For this review, take the finished solid that the model builds, in its own axes (mm). Face numbers are marked on the shaded views. A direction names the side the tool comes from. Give positions to 0.01 mm unless a question says otherwise; leave off trailing zeros. Write each loop counter-clockwise with the first axis right and the second up, starting at its lowest first coordinate (ties: lowest second). Pieces come first, ordered by that corner, then holes. Notation, with made-up numbers: (16, 61) -> (48, 61) arc R22 cw to (48, 69) -> close; hole circle Ø2 at (66, -20). An arc over 180 degrees is marked (long way). Write item = value, one per line.
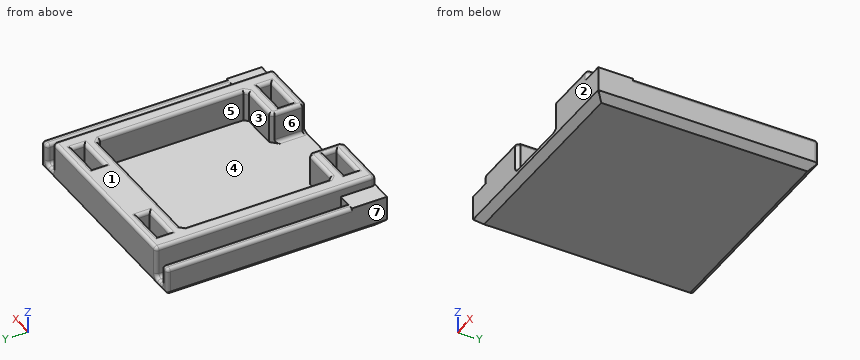
```python
from build123d import *

# Parameters (mm, degrees)
BOSS_EXTRU_2_DEPTH      = 9
ESQUISSE3_W             = 51.8612703
ESQUISSE3_H             = 63
BOSS_EXTRU_3_DEPTH      = 3
ESQUISSE4_W             = 10
ESQUISSE4_H             = 3.4
ENL_V_MAT_EXTRU_1_DEPTH = 7
ESQUISSE5_W             = 3.2
ESQUISSE5_H             = 3
BOSS_EXTRU_4_DEPTH      = 63
CHANFREIN1_SIZE         = 1
CHANFREIN2_SIZE         = 2
CONG_1_R                = 1
CONG_2_R                = 1
CHANFREIN4_SIZE         = 1
CONG_4_R                = 1
CONG_5_R                = 1
ESQUISSE6_W             = 6.7
ESQUISSE6_H             = 1
BOSS_EXTRU_5_DEPTH      = 10


with BuildPart() as part:
    # Esquisse2 → Boss.-Extru.2 (new body)
    with BuildSketch(Plane.XY):
        Polygon((-9.3, -31.5), (-9.3, -21.5), (-21.5, -21.5), (-21.5, 21.5), (21.5, 21.5), (21.5, -21.5), (9.3, -21.5), (9.3, -31.5), (25.93063515, -31.5), (25.93063515, 31.5), (-25.93063515, 31.5), (-25.93063515, -31.5), align=None)
    extrude(amount=BOSS_EXTRU_2_DEPTH)

    # Esquisse3 → Boss.-Extru.3 (add)
    with BuildSketch(Plane(origin=(0, 0, 0), x_dir=(-1, 0, 0), z_dir=(0, 0, -1))):
        Rectangle(ESQUISSE3_W, ESQUISSE3_H)
    extrude(amount=BOSS_EXTRU_3_DEPTH)

    # Esquisse4 → Enlèv. mat.-Extru.1 (cut)
    with BuildSketch(Plane.XY.offset(9)):
        with Locations((-16.5, -26.695538472)):
            Rectangle(ESQUISSE4_W, ESQUISSE4_H)
        with Locations((16.5, -26.695538472)):
            Rectangle(ESQUISSE4_W, ESQUISSE4_H)
        with Locations((16.5, 26.695538472)):
            Rectangle(ESQUISSE4_W, ESQUISSE4_H)
        with Locations((-16.5, 26.695538472)):
            Rectangle(ESQUISSE4_W, ESQUISSE4_H)
    extrude(amount=-ENL_V_MAT_EXTRU_1_DEPTH, mode=Mode.SUBTRACT)

    # Esquisse5 → Boss.-Extru.4 (add)
    with BuildSketch(Plane(origin=(0, 31.5, 0), x_dir=(1, 0, 0), z_dir=(0, 1, 0))):
        Polygon((-29.13063515, 0), (-29.13063515, 3), (-31.63063515, 3), (-31.63063515, -6), (-29.13063515, -6), align=None)
        with Locations((-27.53063515, 1.5)):
            Rectangle(ESQUISSE5_W, ESQUISSE5_H)
        with Locations((27.53063515, 1.5)):
            Rectangle(ESQUISSE5_W, ESQUISSE5_H)
        Polygon((29.13063515, 3), (29.13063515, 0), (29.13063515, -6), (31.63063515, -6), (31.63063515, 3), align=None)
    extrude(amount=-BOSS_EXTRU_4_DEPTH)

    # Chanfrein1
    chanfrein1_edges = [part.edges().sort_by_distance(p)[0] for p in [
        (21.5, -21.5, 4.5),
        (21.5, 21.5, 4.5),
        (-21.5, 21.5, 4.5),
        (-21.5, -21.5, 4.5),
    ]]
    chamfer(chanfrein1_edges, length=CHANFREIN1_SIZE)

    # Chanfrein2
    chanfrein2_edges = [part.edges().sort_by_distance(p)[0] for p in [
        (-31.63063515, 0, -3),
        (31.63063515, 0, -3),
        (0, -31.5, -3),
        (0, 31.5, -3),
    ]]
    chamfer(chanfrein2_edges, length=CHANFREIN2_SIZE)

    # Congé1
    cong_1_edges = [part.edges().sort_by_distance(p)[0] for p in [
        (-25.93063515, 0, 0),
        (-29.13063515, 0, 0),
        (-29.13063515, 0, 6),
        (-31.63063515, 0, 6),
        (25.93063515, 0, 0),
        (29.13063515, 0, 0),
        (29.13063515, 0, 6),
        (31.63063515, 0, 6),
    ]]
    fillet(cong_1_edges, radius=CONG_1_R)

    # Congé2
    cong_2_edges = [part.edges().sort_by_distance(p)[0] for p in [
        (-31.63063515, 31.5, 2),
        (31.63063515, 31.5, 2),
        (30.38063515, -31.5, 6),
        (30.38063515, 31.5, 6),
        (-30.38063515, 31.5, 6),
        (-29.13063515, 31.5, 3),
        (-27.53063515, 31.5, 0),
        (27.53063515, 31.5, 0),
        (29.13063515, 31.5, 3),
        (-31.337741931, 31.5, 5.707106781),
        (-29.423528369, 31.5, 5.707106781),
        (29.423528369, 31.5, 5.707106781),
        (31.337741931, 31.5, 5.707106781),
        (31.63063515, -31.5, 2),
        (-31.63063515, -31.5, 2),
        (29.13063515, -31.5, 3),
        (27.53063515, -31.5, 0),
        (-27.53063515, -31.5, 0),
        (-29.13063515, -31.5, 3),
        (-30.38063515, -31.5, 6),
        (-31.337741931, -31.5, 5.707106781),
        (-29.423528369, -31.5, 5.707106781),
        (29.423528369, -31.5, 5.707106781),
        (31.337741931, -31.5, 5.707106781),
        (28.837741931, 31.5, 0.292893219),
        (28.837741931, -31.5, 0.292893219),
        (26.223528369, 31.5, 0.292893219),
        (26.223528369, -31.5, 0.292893219),
        (-28.837741931, 31.5, 0.292893219),
        (-28.837741931, -31.5, 0.292893219),
        (-26.223528369, 31.5, 0.292893219),
        (-26.223528369, -31.5, 0.292893219),
        (-25.93063515, -31.5, 5),
        (-25.93063515, 31.5, 5),
        (25.93063515, 31.5, 5),
        (25.93063515, -31.5, 5),
    ]]
    fillet(cong_2_edges, radius=CONG_2_R - 0.0001)  # a hair under: the kernel refuses the full size

    # Chanfrein4
    chanfrein4_edges = [part.edges().sort_by_distance(p)[0] for p in [
        (-9.3, -31.5, 4.5),
        (9.3, -31.5, 4.5),
        (9.3, -21.5, 4.5),
        (-9.3, -21.5, 4.5),
    ]]
    chamfer(chanfrein4_edges, length=CHANFREIN4_SIZE)

    # Congé4
    cong_4_edges = [part.edges().sort_by_distance(p)[0] for p in [
        (-21.5, 0, 9),
        (-15.4, -21.5, 9),
        (21.5, 0, 9),
        (0, 21.5, 9),
        (-21, -21, 9),
        (21, -21, 9),
        (21, 21, 9),
        (-21, 21, 9),
        (0, 31.5, 9),
        (-17.615367575, -31.5, 9),
        (-25.93063515, 0, 9),
        (25.93063515, 0, 9),
        (25.63777122, 31.207136071, 9),
        (25.63777122, -31.207136071, 9),
        (-25.63777122, -31.207136071, 9),
        (-25.63777122, 31.207136071, 9),
        (17.615367575, -31.5, 9),
        (9.3, -26.5, 9),
        (-9.3, -26.5, 9),
        (15.4, -21.5, 9),
        (-9.8, -22, 9),
        (9.8, -22, 9),
        (-9.8, -31, 9),
        (9.8, -31, 9),
        (-16.5, 28.395538472, 9),
        (-11.5, 26.695538472, 9),
        (-21.5, 26.695538472, 9),
        (-16.5, 24.995538472, 9),
        (21.5, 26.695538472, 9),
        (16.5, 24.995538472, 9),
        (16.5, 28.395538472, 9),
        (11.5, 26.695538472, 9),
        (16.5, -28.395538472, 9),
        (11.5, -26.695538472, 9),
        (21.5, -26.695538472, 9),
        (16.5, -24.995538472, 9),
        (-21.5, -26.695538472, 9),
        (-16.5, -24.995538472, 9),
        (-16.5, -28.395538472, 9),
        (-11.5, -26.695538472, 9),
    ]]
    fillet(cong_4_edges, radius=CONG_4_R - 0.0001)  # a hair under: the kernel refuses the full size

    # Congé5
    cong_5_edges = [part.edges().sort_by_distance(p)[0] for p in [
        (9.3, -26.5, 0),
        (-9.3, -26.5, 0),
        (9.8, -31, 0),
        (-9.8, -31, 0),
    ]]
    fillet(cong_5_edges, radius=CONG_5_R)

    # Esquisse6 → Boss.-Extru.5 (add)
    with BuildSketch(Plane.XZ.offset(31.5)):
        with BuildLine():
            Line((-24.93063515, 1), (-24.93063515, 5))
            Line((-24.93063515, 5), (-31.63063515, 5))
            Line((-31.63063515, 5), (-31.63063515, -1))
            Line((-31.63063515, -1), (-26.93063515, -1))
            ThreePointArc((-26.93063515, -1), (-25.516421587, -0.414213562), (-24.93063515, 1))
        make_face()
        with Locations((-28.28063515, 5.5)):
            Rectangle(ESQUISSE6_W, ESQUISSE6_H)
        with BuildLine():
            Line((31.63063515, -1), (31.63063515, 5))
            Line((31.63063515, 5), (24.93063515, 5))
            Line((24.93063515, 5), (24.93063515, 1))
            ThreePointArc((24.93063515, 1), (25.516421587, -0.414213562), (26.93063515, -1))
            Line((26.93063515, -1), (31.63063515, -1))
        make_face()
        with Locations((28.28063515, 5.5)):
            Rectangle(ESQUISSE6_W, ESQUISSE6_H)
    extrude(amount=-BOSS_EXTRU_5_DEPTH)


solid = part.part
```
(1) The part is to be moulded in two halves that separate along Y. For the marked faces 1, 2, 3 and 4, say which applies: released by +Y, released by -Y, zero draft, split by the parting line, or undercut.
Answers below:
face_1 = zero draft
face_2 = released by -Y
face_3 = undercut
face_4 = undercut
(2) Take a section at B-B (z = 2.75). Count the separate pieces of the cut face and the enclosed holes in it, plus the area to 3 significant figures.
Answers below:
separate_pieces = 1
enclosed_holes = 4
area = 1,470 mm^2
(3) Take a section at D-D (x = -15.5). Write out the cut boundary in (y, z).
Answers below:
outline = (-31.5, -1) -> (-29.5, -3) -> (29.5, -3) -> (31.5, -1) -> (31.5, 8) arc R1 ccw to (30.5, 9) -> (29.4, 9) arc R1 ccw to (28.4, 8) -> (28.4, 2) -> (25, 2) -> (25, 8) arc R1 ccw to (24, 9) -> (22.5, 9) arc R1 ccw to (21.5, 8) -> (21.5, 0) -> (-21.5, 0) -> (-21.5, 8) arc R1 ccw to (-22.5, 9) -> (-24, 9) arc R1 ccw to (-25, 8) -> (-25, 2) -> (-28.4, 2) -> (-28.4, 8) arc R1 ccw to (-29.4, 9) -> (-30.5, 9) arc R1 ccw to (-31.5, 8) -> close
(4) Tool access review of the marked faces 5, 6 and 7: name each direction out of +Z, -Z, +X, -X, +Y, -Y from which nothing blocks a thin tool from reaching the whole face with its end or side.
Answers below:
face_5 = +Z
face_6 = +Z, -Y
face_7 = +Z, -Z, -X, +Y, -Y
(5) To check wall thickness, follow probe 1 along Y at (x, z) = (13, 3.75); probe 2 along X at (y, z) = (22, 4); probe 3 along X at (y, z) = (-15, 4.5). State the ranges of each line that lie inside material, in increasing order.
Answers below:
probe_1 = -31.5 to -28.4, -25 to -21.5, 21.5 to 25, 28.4 to 31.5
probe_2 = -31.63 to -29.13, -25.93 to 25.93, 29.13 to 31.63
probe_3 = -31.63 to -29.13, -25.93 to -21.5, 21.5 to 25.93, 29.13 to 31.63
(6) Take a section at A-A (x = 3). Write out the cut boundary in (y, z), plus the area to 3 significant figures.
Answers below:
outline = (-31.5, -1) -> (-29.5, -3) -> (29.5, -3) -> (31.5, -1) -> (31.5, 8) arc R1 ccw to (30.5, 9) -> (22.5, 9) arc R1 ccw to (21.5, 8) -> (21.5, 0) -> (-31.5, 0) -> close
area = 275 mm^2
(7) For pin 1 (4 mm diameter, centred on x = -6.5, y = -4.5, fed in from +Z); pin 2 (2.5 mm diameter, centred on x = -14.5, y = 26.5, fed in from +Z); pin 3 (5.5 mm diameter, centred on x = 29.5, y = 4, fed in from +Z), all flat-tipped, find the tip position at first contact; note any pin that passes through.
Answers below:
pin_1 = 0
pin_2 = 2
pin_3 = 6
